Read the model definition and answer for the solid it produces. Units are mm, in the model's axes. Coordinates: 2 decimals unless noted, no trailing zeros. Order: outer loops, then holes, each group sorted by start corner. A loop starts at its lowest first (then second) coordinate and runs counter-clockwise, first axis right, second up. Notation, with made-up numbers: (9, 33.25) -> (29, 33.25) arc R28 cw to (29, 54.25) -> close; hole circle Ø4 at (43.25, 68). An arc over 180 degrees is marked (long way). Answer in a Markdown table with one row per item.
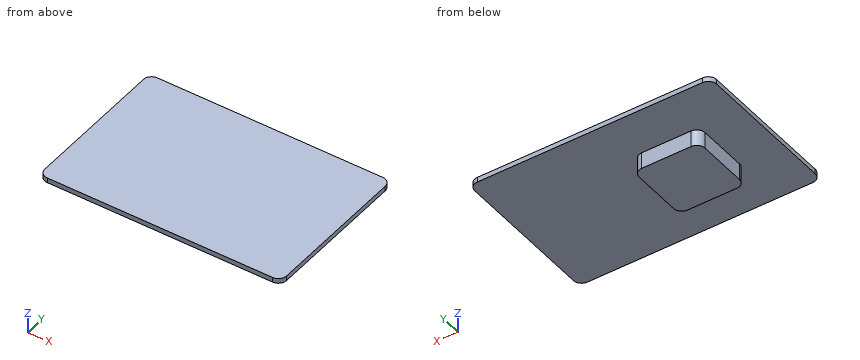
from build123d import *

# Parameters (mm, degrees)
EXTRUDE_1_DEPTH = 30
EXTRUDE_2_DEPTH = 100


with BuildPart() as part:
    # 草图2 → 凸台-拉伸1 (new body)
    with BuildSketch(Plane.XY):
        with BuildLine():
            Line((-1075.548373655, 479.992677665), (293.974322669, 479.992677665))
            ThreePointArc((293.974322669, 479.992677665), (329.329661728, 465.348016724), (343.974322669, 429.992677665))
            Line((343.974322669, 429.992677665), (343.974322669, -429.992677665))
            ThreePointArc((343.974322669, -429.992677665), (329.329661728, -465.348016724), (293.974322669, -479.992677665))
            Line((293.974322669, -479.992677665), (-1075.548373655, -479.992677665))
            ThreePointArc((-1075.548373655, -479.992677665), (-1110.903712715, -465.348016724), (-1125.548373655, -429.992677665))
            Line((-1125.548373655, -429.992677665), (-1125.548373655, 429.992677665))
            ThreePointArc((-1125.548373655, 429.992677665), (-1110.903712715, 465.348016724), (-1075.548373655, 479.992677665))
        make_face()
    extrude(amount=EXTRUDE_1_DEPTH)

    # 草图4 → 凸台-拉伸2 (add)
    with BuildSketch(Plane(origin=(0, 0, 0), x_dir=(-1, 0, 0), z_dir=(0, 0, -1))):
        with BuildLine():
            Line((510, 200), (810, 200))
            ThreePointArc((810, 200), (845.355339059, 185.355339059), (860, 150))
            Line((860, 150), (860, -150))
            ThreePointArc((860, -150), (845.355339059, -185.355339059), (810, -200))
            Line((810, -200), (510, -200))
            ThreePointArc((510, -200), (474.644660941, -185.355339059), (460, -150))
            Line((460, -150), (460, 150))
            ThreePointArc((460, 150), (474.644660941, 185.355339059), (510, 200))
        make_face()
    extrude(amount=EXTRUDE_2_DEPTH)


solid = part.part
Q1. The part is cut by section D-D (y = 389.5). Write down the section's boundary in (x, z), then the cut area to 3 significant figures.
Outcome:
| item | result |
|---|---|
| outline | (-1125.55, 0) -> (343.97, 0) -> (343.97, 30) -> (-1125.55, 30) -> close |
| area | 44,100 mm² |
Q2. The part is cut by section B-B (y = -123.5). Write down the section's boundary in (x, z).
Outcome:
| item | result |
|---|---|
| outline | (-1125.55, 0) -> (-860, 0) -> (-860, -100) -> (-460, -100) -> (-460, 0) -> (343.97, 0) -> (343.97, 30) -> (-1125.55, 30) -> close |
Q3. Consider line 1 (X direction, y = 116.5, z = -94.5); line 2 (Z direction, x = -75, y = -181.5); line 3 (Y direction, x = -670.5, z = -69). Determine where each line is inside the solid, lowest interval first.
Outcome:
| item | result |
|---|---|
| line 1 | -860 to -460 |
| line 2 | 0 to 30 |
| line 3 | -200 to 200 |
Q4. The part is cut by section A-A (z = -59). Write down the section's boundary in (x, y), then the cut area to 3 significant figures.
Outcome:
| item | result |
|---|---|
| outline | (-860, -150) arc R50 ccw to (-810, -200) -> (-510, -200) arc R50 ccw to (-460, -150) -> (-460, 150) arc R50 ccw to (-510, 200) -> (-810, 200) arc R50 ccw to (-860, 150) -> close |
| area | 158,000 mm² |
Q5. The part is cut by section C-C (x = -367). Write down the section's boundary in (y, z).
Outcome:
| item | result |
|---|---|
| outline | (-479.99, 0) -> (479.99, 0) -> (479.99, 30) -> (-479.99, 30) -> close |
Q6. Given pin 1 (5 mm diameter, centred on x = -485.5, z = -75.5, fed in from -Y); pin 2 (1 mm diameter, centred on x = -873.5, y = -276.5, fed in from -Z), each flat-ended and moving along its own axis, determine where each tip first touches the part or whether it passes through.
Outcome:
| item | result |
|---|---|
| pin 1 | y = -194.9 |
| pin 2 | z = 0 |
